```python
from build123d import *
from OCP.BRepFilletAPI import BRepFilletAPI_MakeChamfer

# Parameters (mm, degrees)
SKETCH1_W           = 17.5
SKETCH1_H           = 16.5
BOSS_EXTRUDE1_DEPTH = 3
SKETCH2_W           = 2.707061395
SKETCH2_H           = 1.1
SKETCH2_W_2         = 2.5
CUT_EXTRUDE1_DEPTH  = 14.5
CHAMFER1_SIZE       = 1.5
CHAMFER1_SIZE2      = 3.216760381
CHAMFER2_SIZE       = 1
CHAMFER2_SIZE2      = 0.577350269
SKETCH3_W           = 12.292938605
SKETCH3_H           = 15.922649731
BOSS_EXTRUDE2_DEPTH = 8
SKETCH4_W           = 12.292938605
SKETCH4_H           = 3
BOSS_EXTRUDE3_DEPTH = 120
CHAMFER3_SIZE       = 4
CHAMFER3_SIZE2      = 8.578027682
SKETCH5_W           = 12.292938605
SKETCH5_H           = 0.577350269
BOSS_EXTRUDE4_DEPTH = 10
SKETCH6_R           = 12
BOSS_EXTRUDE7_DEPTH = 15
CUT_EXTRUDE3_DEPTH  = 15
SKETCH10_R          = 1
CUT_EXTRUDE4_DEPTH  = 15
CHAMFER5_SIZE       = 2
CHAMFER5_SIZE2      = 2.054853594
SKETCH11_W          = 8.292938605
SKETCH11_H          = 2
CUT_EXTRUDE5_DEPTH  = 1.5


with BuildPart() as part:
    # Sketch1 → Boss-Extrude1 (new body)
    with BuildSketch(Plane(origin=(0, 0, 0), x_dir=(1, 0, 0), z_dir=(0, 1, 0))):
        with Locations((-7.963643791, 7.469362745)):
            Rectangle(SKETCH1_W, SKETCH1_H)
    extrude(amount=BOSS_EXTRUDE1_DEPTH)

    # Sketch2 → Cut-Extrude1 (cut)
    with BuildSketch(Plane.XY.offset(0.780637255)):
        with Locations((-15.360113094, 2.45)):
            Rectangle(SKETCH2_W, SKETCH2_H)
        with Locations((-0.463643791, 2.45)):
            Rectangle(SKETCH2_W_2, SKETCH2_H)
    extrude(amount=-CUT_EXTRUDE1_DEPTH, mode=Mode.SUBTRACT)

    # Chamfer1
    chamfer1_edges = [part.edges().sort_by_distance(p)[0] for p in [
        (-15.360113093, 1.9, 0.780637255),
        (-0.463643791, 1.9, 0.780637255),
    ]]
    chamfer1_side = [part.faces().sort_by_distance(p)[0] for p in [
        (-7.933712225, 1.383662189, 0.780637255),
    ]]
    chamfer(chamfer1_edges, length=CHAMFER1_SIZE, length2=CHAMFER1_SIZE2, reference=chamfer1_side[0])

    # Chamfer2
    chamfer2_edges = [part.edges().sort_by_distance(p)[0] for p in [
        (-7.963643791, 3, -15.719362745),
    ]]
    chamfer2_side = [part.faces().sort_by_distance(p)[0] for p in [
        (-7.963643791, 1.5, -15.719362745),
    ]]
    chamfer(chamfer2_edges, length=CHAMFER2_SIZE, length2=CHAMFER2_SIZE2, reference=chamfer2_side[0])

    # Sketch3 → Boss-Extrude2 (add)
    with BuildSketch(Plane(origin=(0, 3, 0), x_dir=(1, 0, 0), z_dir=(0, 1, 0))):
        with Locations((-7.860113094, 7.180687611)):
            Rectangle(SKETCH3_W, SKETCH3_H)
    extrude(amount=BOSS_EXTRUDE2_DEPTH)

    # Sketch4 → Boss-Extrude3 (add)
    with BuildSketch(Plane.XY.offset(0.780637255)):
        with Locations((-7.860113094, 9.5)):
            Rectangle(SKETCH4_W, SKETCH4_H)
    extrude(amount=BOSS_EXTRUDE3_DEPTH)

    # Chamfer3
    chamfer3_edges = [part.edges().sort_by_distance(p)[0] for p in [
        (-7.860113093, 8, 0.780637255),
    ]]
    chamfer3_side = [part.faces().sort_by_distance(p)[0] for p in [
        (-7.867329476, 3.921188666, 0.780637255),
    ]]
    chamfer(chamfer3_edges, length=CHAMFER3_SIZE, length2=CHAMFER3_SIZE2, reference=chamfer3_side[0])

    # Sketch5 → Boss-Extrude4 (add)
    with BuildSketch(Plane(origin=(0, 11, 0), x_dir=(1, 0, 0), z_dir=(0, 1, 0))):
        with Locations((-7.860113094, 15.430687611)):
            Rectangle(SKETCH5_W, SKETCH5_H)
    extrude(amount=-BOSS_EXTRUDE4_DEPTH)

    # Sketch6 → Boss-Extrude7 (add)
    with BuildSketch(Plane(origin=(0, 0, -15.719362745), x_dir=(-1, 0, 0), z_dir=(0, 0, -1))):
        with BuildLine():
            Line((1.713643791, 11), (14.006582396, 11))
            Line((14.006582396, 11), (14.006582396, 12.317130596))
            ThreePointArc((14.006582396, 12.317130596), (7.860113093, 41), (1.713643791, 12.317130596))
            Line((1.713643791, 12.317130596), (1.713643791, 11))
        make_face()
        with Locations((7.860113093, 26)):
            Circle(SKETCH6_R, mode=Mode.SUBTRACT)
    extrude(amount=-BOSS_EXTRUDE7_DEPTH)

    # Sketch7 → Cut-Extrude3 (cut)
    with BuildSketch(Plane(origin=(0, 11, 0), x_dir=(1, 0, 0), z_dir=(0, 1, 0))):
        Polygon((-11.006582396, -120.780637255), (-14.006582396, -6.957338355), (-14.006582396, -120.780637255), align=None)
        Polygon((-4.713643791, -120.780637255), (-1.713643791, -120.780637255), (-1.713643791, -6.957338355), align=None)
    extrude(amount=-CUT_EXTRUDE3_DEPTH, mode=Mode.SUBTRACT)

    # Sketch10 → Cut-Extrude4 (cut)
    with BuildSketch(Plane(origin=(0, 11, 0), x_dir=(1, 0, 0), z_dir=(0, 1, 0))):
        with Locations(Location((-7.860113093, -117.478934199, 0), (0, 0, 270))):
            Circle(SKETCH10_R)
    extrude(amount=-CUT_EXTRUDE4_DEPTH, mode=Mode.SUBTRACT)

    # Chamfer5: one chamfer whose edges measure the first distance from different faces: ONE call of the kernel's chamfer builder (chamfer() names one face for all edges)
    chamfer5_edges_1 = [part.edges().sort_by_distance(p)[0] for p in [
        (-11.006582396, 9.5, 120.780637255),
    ]]
    chamfer5_side_1 = [part.faces().sort_by_distance(p)[0] for p in [
        (-7.860113093, 9.5, 120.780637255),
    ]]
    chamfer5_edges_2 = [part.edges().sort_by_distance(p)[0] for p in [
        (-4.713643791, 9.5, 120.780637255),
    ]]
    chamfer5_side_2 = [part.faces().sort_by_distance(p)[0] for p in [
        (-3.207843821, 9.492653469, 63.64893058),
    ]]
    chamfer5 = BRepFilletAPI_MakeChamfer(part.part.solid().wrapped)
    for e in chamfer5_edges_1:
        chamfer5.Add(CHAMFER5_SIZE, CHAMFER5_SIZE2, e.wrapped, chamfer5_side_1[0].wrapped)  # the first distance lies on this face
    for e in chamfer5_edges_2:
        chamfer5.Add(CHAMFER5_SIZE, CHAMFER5_SIZE2, e.wrapped, chamfer5_side_2[0].wrapped)  # the first distance lies on this face
    add(Compound.cast(chamfer5.Shape()), mode=Mode.REPLACE)

    # Sketch11 → Cut-Extrude5 (cut)
    with BuildSketch(Plane.XY.offset(0.780637255)):
        with Locations((-7.860113094, 1)):
            Rectangle(SKETCH11_W, SKETCH11_H)
    extrude(amount=-CUT_EXTRUDE5_DEPTH, mode=Mode.SUBTRACT)


solid = part.part
```
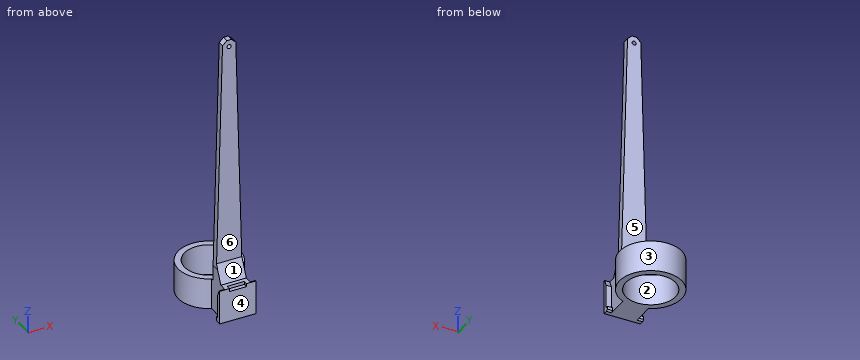
Could you check a few things on this model? Use its own coordinates, in mm. Face numbers are marked on the shaded views. A direction names the side the tool comes from. Round coordinates to 2 decimals unless told otherwise and drop trailing zeros. Write each loop counter-clockwise with the first axis right and the second up, starting at its lowest first coordinate (ties: lowest second). Pieces come first, ordered by that corner, then holes. Notation, with made-up numbers: M 50.25,70 L 61.25,70 A31 cw 61.25,102 Z; hole C 69,-18 d1. An arc over 180 degrees is marked long. Answer in a Markdown table with one row per item. Add a question column.
Q1. On a 3-axis mill with a long thin cutter (end or side, diameter ignored), from which of +Z, -Z, +X, -X, +Y, -Y can I reach the whole of each face in a straight line? I mean the marked faces 4, 5 and 6. Say none if no direction works.
Q2. Will these pins go through, and if not, where does the flat tip stop? pin 1 Ø0.5 at (x, y) = (-1, 2.5) entering from +Z; pin 2 Ø0.7 at (x, z) = (-15.5, -14) entering from +Y; pin 3 Ø6 at (x, z) = (-13, 83) entering from +Y.
Q3. If I drill on line 1 (Y direction, x = -5, z = -6); line 2 (X direction, y = 7.5, z = -4); line 3 (Y direction, x = -13, z = -8.5), over which ranges is the centre line in solid material (lowest first)? Write a range as from..to.
Q4. Imagine slicing it at B-B (y = 36). Please give me the cut outline in (x, z).
Q5. If we mould it in two halves opening along X, with no side actions, what happens to the marked faces 1, 2 and 3? For each: +X half, -X half, draft (parallel to the pull), parting line (faces both ways), or undercut.
Q6. Imagine slicing it at D-D (z = 90). Please give me the cut outline in (x, y).
Q7. Imagine slicing it at A-A (y = 26). Please give me the cut outline in (x, z).
Q8. Imagine slicing it at C-C (z = 57). Please give me the cut outline in (x, y), then the cut area to 3 significant figures.
Values:
| question | item | result |
|---|---|---|
| 1 | face 4 | +Z, -Z, +X, -X, -Y |
| 1 | face 5 | +Z, +X, -X, +Y |
| 1 | face 6 | +Z, +X, -X, -Y |
| 2 | pin 1 | z = -13.72 |
| 2 | pin 2 | y = 39.11 |
| 2 | pin 3 | y = 11 |
| 3 | line 1 | 0..14.35, 37.65..40.72 |
| 3 | line 2 | -14.01..-1.71 |
| 3 | line 3 | 0..15.16, 36.84..40.09 |
| 4 | outline | M -19.04,-15.72 L -14.49,-15.72 L -14.49,-0.72 L -19.04,-0.72 Z; M -1.23,-15.72 L 3.32,-15.72 L 3.32,-0.72 L -1.23,-0.72 Z |
| 5 | face 1 | draft |
| 5 | face 2 | undercut |
| 5 | face 3 | parting line |
| 6 | outline | M -11.82,8 L -3.9,8 L -3.9,11 L -11.82,11 Z |
| 7 | outline | M -22.86,-15.72 L -19.86,-15.72 L -19.86,-0.72 L -22.86,-0.72 Z; M 4.14,-15.72 L 7.14,-15.72 L 7.14,-0.72 L 4.14,-0.72 Z |
| 8 | outline | M -12.69,8 L -3.03,8 L -3.03,11 L -12.69,11 Z |
| 8 | area | 29.0 mm^2 |
